For this review, take the finished solid that the model builds, in its own axes (mm). A direction names the side the tool comes from. Give positions to 0.01 mm unless a question says otherwise; leave off trailing zeros. Order: outer loops, then holes, each group sorted by start corner. A loop starts at its lowest first (then second) coordinate and runs counter-clockwise, first axis right, second up.
from build123d import *

# Parameters (mm, degrees)
F0_R     = 2.4
F1_DEPTH = 15
F3_DEPTH = 25


with BuildPart() as f1:
    # F0 (on Front) → F1 (new body)
    with BuildSketch(Plane.XZ):
        Polygon((16.165808, 28), (-16.165808, 28), (-32.331615, 0), (-16.165808, -28), (16.165808, -28), (32.331615, 0), align=None)
        with Locations((-11.9075, -20.624395)):
            Circle(F0_R, mode=Mode.SUBTRACT)
        with Locations((11.9075, -20.624395)):
            Circle(F0_R, mode=Mode.SUBTRACT)
        with Locations((-23.815, 0)):
            Circle(F0_R, mode=Mode.SUBTRACT)
        with Locations((-11.9075, 20.624395)):
            Circle(F0_R, mode=Mode.SUBTRACT)
        with Locations((23.815, 0)):
            Circle(F0_R, mode=Mode.SUBTRACT)
        with Locations((11.9075, 20.624395)):
            Circle(F0_R, mode=Mode.SUBTRACT)
    extrude(amount=F1_DEPTH)

    # F2 (on face) → F3 (cut)
    with BuildSketch(Plane.XZ.offset(15)):
        with BuildLine():
            ThreePointArc((-6.913185, -8.75), (-3.76319, -12.31774), (0.721978, -10.725728))
            ThreePointArc((0.721978, -10.725728), (9.500181, -5.03081), (9.277499, 5.430516))
            ThreePointArc((9.277499, 5.430516), (6.963643, 10.700233), (1.208341, 10.681873))
            ThreePointArc((1.208341, 10.681873), (-2.697223, 10.406127), (-6.244998, 8.75))
            Line((-6.244998, 8.75), (-18.244998, 8.75))
            Line((-18.244998, 8.75), (-18.244998, -8.75))
            Line((-18.244998, -8.75), (-6.913185, -8.75))
        make_face()
    extrude(amount=-F3_DEPTH, mode=Mode.SUBTRACT)


solid = f1.part
1) Tool access review of faces 1 (the face through (24.362, -7.395, 13.804)), 2 (the face through (-12, -8, 8.75)): name each direction out of +Z, -Z, +X, -X, +Y, -Y from which nothing blocks a thin tool from reaching the whole face with its end or side.
Answer sheet:
face 1: +Z, +X, +Y, -Y
face 2: +Y, -Y
2) We need section B-B on z = -9.5. Give the boundary of the cut face in (x, y).
Answer sheet:
outline: (-26.85, -15) - (-6.75, -15) - (-6.75, 0) - (-26.85, 0) - close; (5.03, -15) - (26.85, -15) - (26.85, 0) - (5.03, 0) - close
3) We need section C-C on x = -1. Give the boundary of the cut face in (y, z), then the cut area to 3 significant figures.
Answer sheet:
outline: (-15, -28) - (0, -28) - (0, -12.1) - (-15, -12.1) - close; (-15, 10.7) - (0, 10.7) - (0, 28) - (-15, 28) - close
area: 498 mm2
4) We need section D-D on y = -13. Count the separate pieces of the cut face and the enclosed holes in it, then the cut area to 3 significant figures.
Answer sheet:
separate pieces: 1
enclosed holes: 7
area: 2,060 mm2
5) To check wall thickness, follow line 1 (X direction, y = -12, z = -1.5) (1 decimal); line 2 (X direction, y = -6.5, z = -19); line 3 (X direction, y = -6.75, z = 22). State the ranges of each line that lie inside material, in increasing order.
Answer sheet:
line 1: x = -31.5 to -25.7, -21.9 to -18.2, 10.6 to 21.9, 25.7 to 31.5
line 2: x = -21.36 to -13.67, -10.14 to 10.14, 13.67 to 21.36
line 3: x = -19.63 to -13.87, -9.94 to 9.94, 13.87 to 19.63
6) We need section A-A on x = -12. Give the boundary of the cut face in (y, z).
Answer sheet:
outline: (-15, -28) - (0, -28) - (0, -23.02) - (-15, -23.02) - close; (-15, -18.23) - (0, -18.23) - (0, -8.75) - (-15, -8.75) - close; (-15, 8.75) - (0, 8.75) - (0, 18.23) - (-15, 18.23) - close; (-15, 23.02) - (0, 23.02) - (0, 28) - (-15, 28) - close
7) Clearance check with flat-ended pins moving along their axes: pin 1 (3 mm diameter, centred on y = -3.5, z = 19, fed in from -X); pin 2 (4 mm diameter, centred on y = -5, z = -18.5, fed in from +X); pin 3 (2 mm diameter, centred on x = -23, y = -9.5, fed in from -Z). State where each tip first meets the part, or that it passes through.
Answer sheet:
pin 1: stops at x = -22.23
pin 2: stops at x = 22.81
pin 3: stops at z = -17.89
8) Draft analysis for pull direction X (two halves, no side actions). For faces 3 (the face through (-18.245, -8, 0)), 4 (the face through (0, -7, 28)), 5 (the face through (-24.136, -7.395, 14.196)), state which applies: +X half, -X half, draft (parallel to the pull), parting line (faces both ways), or undercut.
Answer sheet:
face 3: undercut
face 4: draft
face 5: -X half
